For this review, use the dimensioned drawing (mm, ordinates from the lowest corner) and the shaded views. Coordinates: 2 decimals unless noted, no trailing zeros. Write each loop counter-clockwise with the first axis right and the second up, starting at its lowest first coordinate (ties: lowest second). Pieces come first, ordered by that corner, then holes. Notation, with made-up numbers: (-36.75, 27.25) -> (-18.75, 27.25) arc R21 ccw to (-18.75, 64.25) -> close; hole circle Ø11 at (17, 73.25). An arc over 180 degrees is marked (long way). Return JSON: item names as keys, results as strings. Group by question number.
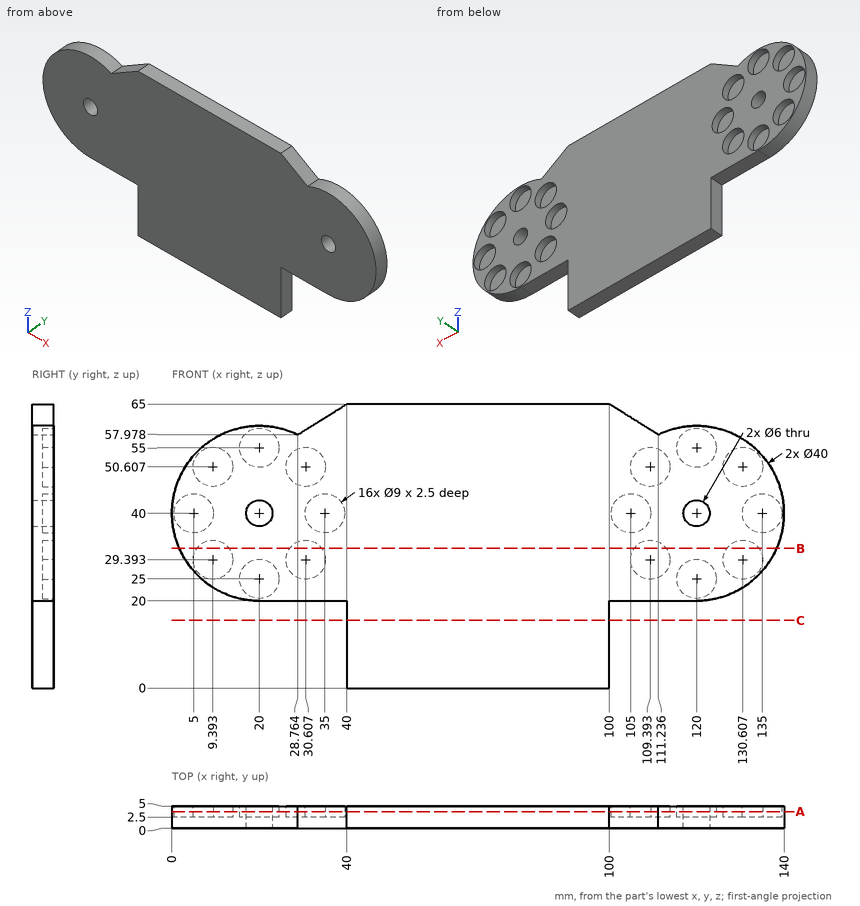
Q1. We need section A-A on y = 3.75. State how many separate pieces and enclosed holes the cut face has, plus the area to 3 significant figures.
Q2. For P1, Ø7, axis at x = 20, z = 55, coming from the +Y side; P2, Ø2, axis at y = 1.5, z = 36.5, coming from the +X side; P3, Ø2.5, axis at y = 3.5, z = 13.5, coming from the -X side, all flat-tipped, find the tip position at first contact; note any pin that passes through.
Q3. Wall thickness on L1, parallel to Z at x = 20, y = 4.2; L2, parallel to X at y = 2.45, z = 40; L3, parallel to X at y = 3.4, z = 56 (1 decimal): over which ranges is each line inside the solid? List them lowest first.
Q4. We need section B-B on z = 32. Write out the cut boundary in (x, y) (1 decimal), plus the area to 3 significant figures.
Q5. We need section C-C on z = 15.5. Write out the cut boundary in (x, y), plus the area to 3 significant figures.
Findings below:
{
 "1": {"separate pieces": "1", "enclosed holes": "18", "area": "5,700 mm^2"},
 "2": {"P1": "stops at y = 2.5", "P2": "stops at x = 139.84", "P3": "stops at x = 40"},
 "3": {"L1": "z = 20 to 20.5, 29.5 to 37, 43 to 50.5, 59.5 to 60", "L2": "x = 0 to 17, 23 to 117, 123 to 140", "L3": "x = 8 to 15.6, 24.4 to 115.6, 124.4 to 132"},
 "4": {"outline": "(1.7, 0) -> (138.3, 0) -> (138.3, 5) -> (134.3, 5) -> (134.3, 2.5) -> (126.9, 2.5) -> (126.9, 5) -> (113.1, 5) -> (113.1, 2.5) -> (105.7, 2.5) -> (105.7, 5) -> (34.3, 5) -> (34.3, 2.5) -> (26.9, 2.5) -> (26.9, 5) -> (13.1, 5) -> (13.1, 2.5) -> (5.7, 2.5) -> (5.7, 5) -> (1.7, 5) -> close", "area": "610 mm^2"},
 "5": {"outline": "(40, 0) -> (100, 0) -> (100, 5) -> (40, 5) -> close", "area": "300 mm^2"}
}
